from build123d import *

# Parameters (mm, degrees)
SKETCH1_W           = 60
SKETCH1_H           = 36
SKETCH1_R           = 2
BOSS_EXTRUDE1_DEPTH = 6.5
SKETCH2_W           = 9.5
SKETCH2_H           = 20
SKETCH2_H_2         = 21
BOSS_EXTRUDE2_DEPTH = 22
CUT_EXTRUDE1_REACH  = 71.572
SKETCH3_R           = 1.5
CUT_EXTRUDE2_DEPTH  = 3
LPATTERN1_COUNT     = 2
LPATTERN1_PITCH     = 32
FILLET1_R           = 1
SKETCH6_W           = 8
SKETCH6_H           = 3
CUT_EXTRUDE3_DEPTH  = 76.181447179


with BuildPart() as part:
    # Sketch1 → Boss-Extrude1 (new body)
    with BuildSketch(Plane.XY):
        with Locations((30, -18)):
            Rectangle(SKETCH1_W, SKETCH1_H)
        with Locations(Location((14, -4.5, 0), (0, 0, 180))):
            Circle(SKETCH1_R, mode=Mode.SUBTRACT)
        with Locations(Location((46, -4.5, 0), (0, 0, 180))):
            Circle(SKETCH1_R, mode=Mode.SUBTRACT)
    extrude(amount=BOSS_EXTRUDE1_DEPTH)

    # Sketch2 → Boss-Extrude2 (add)
    with BuildSketch(Plane.XZ.offset(36)):
        with Locations((4.75, 16.5)):
            Rectangle(SKETCH2_W, SKETCH2_H)
        with Locations((55.25, 17)):
            Rectangle(SKETCH2_W, SKETCH2_H_2)
    extrude(amount=-BOSS_EXTRUDE2_DEPTH)

    # Sketch3 → Cut-Extrude1 (cut, up to next)
    with BuildSketch(Plane(origin=(0, -14, 0), x_dir=(1, 0, 0), z_dir=(0, 1, 0)), mode=Mode.PRIVATE) as cut_extrude1_sk1:
        with Locations(Location((6, -11.5, 0), (0, 0, 270))):
            Circle(SKETCH3_R)
    cut_extrude1_tool1 = extrude(cut_extrude1_sk1.sketch, amount=-CUT_EXTRUDE1_REACH, mode=Mode.PRIVATE) & part.part
    # Sketch3 → Cut-Extrude1 (cut, up to next)
    with BuildSketch(Plane(origin=(0, -14, 0), x_dir=(1, 0, 0), z_dir=(0, 1, 0)), mode=Mode.PRIVATE) as cut_extrude1_sk2:
        with Locations(Location((54, -11.5, 0), (0, 0, 270))):
            Circle(SKETCH3_R)
    cut_extrude1_tool2 = extrude(cut_extrude1_sk2.sketch, amount=-CUT_EXTRUDE1_REACH, mode=Mode.PRIVATE) & part.part
    # Sketch3 → Cut-Extrude1 (cut, up to next)
    with BuildSketch(Plane(origin=(0, -14, 0), x_dir=(1, 0, 0), z_dir=(0, 1, 0)), mode=Mode.PRIVATE) as cut_extrude1_sk3:
        with Locations(Location((54, -21.5, 0), (0, 0, 270))):
            Circle(SKETCH3_R)
    cut_extrude1_tool3 = extrude(cut_extrude1_sk3.sketch, amount=-CUT_EXTRUDE1_REACH, mode=Mode.PRIVATE) & part.part
    # Sketch3 → Cut-Extrude1 (cut, up to next)
    with BuildSketch(Plane(origin=(0, -14, 0), x_dir=(1, 0, 0), z_dir=(0, 1, 0)), mode=Mode.PRIVATE) as cut_extrude1_sk4:
        with Locations(Location((6, -21.5, 0), (0, 0, 270))):
            Circle(SKETCH3_R)
    cut_extrude1_tool4 = extrude(cut_extrude1_sk4.sketch, amount=-CUT_EXTRUDE1_REACH, mode=Mode.PRIVATE) & part.part
    add(cut_extrude1_tool1.solids().sort_by_distance((6, -14, 11.5))[0], mode=Mode.SUBTRACT)
    add(cut_extrude1_tool2.solids().sort_by_distance((54, -14, 11.5))[0], mode=Mode.SUBTRACT)
    add(cut_extrude1_tool3.solids().sort_by_distance((54, -14, 21.5))[0], mode=Mode.SUBTRACT)
    add(cut_extrude1_tool4.solids().sort_by_distance((6, -14, 21.5))[0], mode=Mode.SUBTRACT)

    # Sketch4 → Cut-Extrude2 (cut)
    with BuildSketch(Plane.XY.offset(6.5)):
        Polygon((11.979274058, -1), (9.958548116, -4.5), (11.979274058, -8), (16.020725942, -8), (18.041451884, -4.5), (16.020725942, -1), align=None)
    cut_extrude2 = extrude(amount=-CUT_EXTRUDE2_DEPTH, mode=Mode.SUBTRACT)

    # LPattern1: Cut-Extrude2 ×2
    with Locations(*[(i * LPATTERN1_PITCH, 0, 0) for i in range(1, LPATTERN1_COUNT)]):
        add(cut_extrude2, mode=Mode.SUBTRACT)

    # Fillet1
    fillet1_edges = [part.edges().sort_by_distance(p)[0] for p in [
        (0, -25, 26.5),
        (9.5, -25, 26.5),
        (9.5, -25, 6.5),
        (60, -25, 27.5),
        (50.5, -25, 6.5),
        (50.5, -25, 27.5),
        (60, -18, 0),
        (0, -18, 0),
    ]]
    fillet(fillet1_edges, radius=FILLET1_R)

    # Sketch6 → Cut-Extrude3 (cut, through all)
    with BuildSketch(Plane(origin=(60, 0, 0), x_dir=(0, 0, -1), z_dir=(1, 0, 0))):
        with Locations((-16.5, -34.5)):
            Rectangle(SKETCH6_W, SKETCH6_H)
    extrude(amount=-CUT_EXTRUDE3_DEPTH, mode=Mode.SUBTRACT)


solid = part.part
The listing builds one solid part. Answer for the finished solid, in the listing's coordinates (mm). A direction names the side the tool comes from. Round coordinates to 2 decimals unless told otherwise and drop trailing zeros. Write each loop counter-clockwise with the first axis right and the second up, starting at its lowest first coordinate (ties: lowest second). Pieces come first, ordered by that corner, then holes. Notation, with made-up numbers: (-17.75, -12.75) - (10.25, -12.75) arc R13 cw to (10.25, -3.75) - close; hole circle Ø8 at (5, 8.5). An arc over 180 degrees is marked (long way). Use a Markdown table: item, result. Add a question column.
1. For a pull along X with two mould halves and no side action, classify faces 5 (the face through (0, -22, 13)), 6 (the face through (2, -35, 20.5)), 7 (the face through (17, -6.3, 5)) as +X half, -X half, draft (parallel to the pull), parting line (faces both ways), or undercut.
2. The part is cut by section C-C (y = -27.5). Write down the section's boundary in (x, z).
3. Flat-ended cylindrical pins translate along their axes: P1, Ø4, axis at x = 54, z = 11.5, coming from the +Y side; P2, Ø4, axis at x = 42.5, y = -31, coming from the +Z side; P3, Ø2, axis at x = 47.5, y = -6, coming from the +Z side. Find the tip coordinate at first contact, or state that the pin passes through.
4. The part is cut by section B-B (x = 54). Write down the section's boundary in (y, z).
5. The part is cut by section A-A (z = 24.5). Write down the section's boundary in (x, y).
6. A tool of negligible diameter and unlimited length cuts with its end or side. For faces 1 (the face through (30, -14, 6.5)), 2 (the face through (55, -33, 17)), 3 (the face through (50.5, -25, 17)), 4 (the face through (11, -2.7, 5)), from which of +Z, -Z, +X, -X, +Y, -Y can it reach the whole face along a straight path? Write none if from no direction.
7. The part is cut by section D-D (z = 5.25). Write down the section's boundary in (x, y).
8. Consider line 1 (X direction, y = -26, z = 21.5); line 2 (Z direction, x = 54, y = -22); line 3 (X direction, y = -4.5, z = 1.6). Determine where each line is inside the solid, lowest interval first.
Reported:
| question | item | result |
|---|---|---|
| 1 | face 5 | -X half |
| 1 | face 6 | draft |
| 1 | face 7 | undercut |
| 2 | outline | (0, 1) arc R1 ccw to (1, 0) - (59, 0) arc R1 ccw to (60, 1) - (60, 26.5) arc R1 ccw to (59, 27.5) - (51.5, 27.5) arc R1 ccw to (50.5, 26.5) - (50.5, 7.5) arc R1 cw to (49.5, 6.5) - (10.5, 6.5) arc R1 cw to (9.5, 7.5) - (9.5, 25.5) arc R1 ccw to (8.5, 26.5) - (1, 26.5) arc R1 ccw to (0, 25.5) - close; hole circle Ø3 at (6, 11.5); hole circle Ø3 at (6, 21.5); hole circle Ø3 at (54, 11.5); hole circle Ø3 at (54, 21.5) |
| 3 | P1 | y = -14 |
| 3 | P2 | z = 6.5 |
| 3 | P3 | z = 3.5 |
| 4 | outline | (-36, 0) - (0, 0) - (0, 6.5) - (-14, 6.5) - (-14, 10) - (-36, 10) - close; (-36, 23) - (-14, 23) - (-14, 27.5) - (-36, 27.5) - close; (-33, 13) - (-14, 13) - (-14, 20) - (-33, 20) - close |
| 5 | outline | (0, -36) - (9.5, -36) - (9.5, -14) - (0, -14) - close; (50.5, -36) - (60, -36) - (60, -14) - (50.5, -14) - close |
| 6 | face 1 | +Z, +Y |
| 6 | face 2 | +X, -X, -Y |
| 6 | face 3 | +Z, +Y, -Y |
| 6 | face 4 | +Z |
| 7 | outline | (0, -36) - (60, -36) - (60, 0) - (0, 0) - close; hole (9.96, -4.5) - (11.98, -8) - (16.02, -8) - (18.04, -4.5) - (16.02, -1) - (11.98, -1) - close; hole (41.96, -4.5) - (43.98, -8) - (48.02, -8) - (50.04, -4.5) - (48.02, -1) - (43.98, -1) - close |
| 8 | line 1 | 0 to 4.5, 7.5 to 9.5, 50.5 to 52.5, 55.5 to 60 |
| 8 | line 2 | 0 to 10, 13 to 20, 23 to 27.5 |
| 8 | line 3 | 0 to 12, 16 to 44, 48 to 60 |
